Check sheet for the modelled part. Datum: model origin and axes. Units: mm. A direction names the side the tool comes from. Round coordinates to 2 decimals unless told otherwise and drop trailing zeros. Loops run counter-clockwise (first coordinate to the right, second up) from the corner with the lowest first, then second, coordinate; pieces in that order, holes last. Notation, with made-up numbers: (85, 54) - (116, 54) arc R20 ccw to (116, 74) - close; hole circle Ø1 at (2.25, 54). An arc over 180 degrees is marked (long way). Put each result on its own line as item: value. Start each with the question number.
```python
from build123d import *

# Parameters (mm, degrees)
F0_R     = 12.7
F1_DEPTH = 6.35


with BuildPart() as f1:
    # F0 (on Top) → F1 (new body)
    with BuildSketch(Plane.XY):
        with BuildLine():
            Line((22.45064, 22.45064), (37.34271, 7.55857))
            ThreePointArc((37.34271, 7.55857), (33.570952, 18.016692), (26.940768, 26.940768))
            Line((26.940768, 26.940768), (17.960512, 26.940768))
            Line((17.960512, 26.940768), (22.45064, 22.45064))
        make_face()
        with BuildLine():
            ThreePointArc((-37.34271, -7.55857), (-33.570952, -18.016692), (-26.940768, -26.940768))
            Line((-26.940768, -26.940768), (-17.960512, -26.940768))
            Line((-17.960512, -26.940768), (-22.45064, -22.45064))
            Line((-22.45064, -22.45064), (-37.34271, -7.55857))
        make_face()
        with BuildLine():
            ThreePointArc((7.159566, -37.421259), (17.657349, -33.761339), (26.651684, -27.226783))
            Line((26.651684, -27.226783), (26.747534, -18.247039))
            Line((26.747534, -18.247039), (22.209737, -22.688986))
            Line((22.209737, -22.688986), (7.159566, -37.421259))
        make_face()
        with BuildLine():
            Line((-22.45064, 22.45064), (-7.55857, 37.34271))
            ThreePointArc((-7.55857, 37.34271), (-18.016692, 33.570952), (-26.940768, 26.940768))
            Line((-26.940768, 26.940768), (-26.940768, 17.960512))
            Line((-26.940768, 17.960512), (-22.45064, 22.45064))
        make_face()
        with BuildLine():
            Line((31.75, 6.35), (38.1, 0))
            ThreePointArc((38.1, 0), (37.910205, 3.798206), (37.34271, 7.55857))
            Line((37.34271, 7.55857), (22.45064, 22.45064))
            Line((22.45064, 22.45064), (17.960512, 26.940768))
            Line((17.960512, 26.940768), (26.940768, 26.940768))
            ThreePointArc((26.940768, 26.940768), (24.120826, 29.4923), (21.060567, 31.75))
            Line((21.060567, 31.75), (0, 31.75))
            Line((0, 31.75), (-6.35, 31.75))
            Line((-6.35, 31.75), (0, 38.1))
            ThreePointArc((0, 38.1), (-3.798206, 37.910205), (-7.55857, 37.34271))
            Line((-7.55857, 37.34271), (-22.45064, 22.45064))
            Line((-22.45064, 22.45064), (-26.940768, 17.960512))
            Line((-26.940768, 17.960512), (-26.940768, 26.940768))
            ThreePointArc((-26.940768, 26.940768), (-29.4923, 24.120826), (-31.75, 21.060567))
            Line((-31.75, 21.060567), (-31.75, 0))
            Line((-31.75, 0), (-31.75, -6.35))
            Line((-31.75, -6.35), (-38.1, 0))
            ThreePointArc((-38.1, 0), (-37.910205, -3.798206), (-37.34271, -7.55857))
            Line((-37.34271, -7.55857), (-22.45064, -22.45064))
            Line((-22.45064, -22.45064), (-17.960512, -26.940768))
            Line((-17.960512, -26.940768), (-26.940768, -26.940768))
            ThreePointArc((-26.940768, -26.940768), (-24.120826, -29.4923), (-21.060567, -31.75))
            Line((-21.060567, -31.75), (0, -31.75))
            Line((0, -31.75), (6.35, -31.75))
            Line((6.35, -31.75), (0, -38.1))
            ThreePointArc((0, -38.1), (3.595834, -37.929935), (7.159566, -37.421259))
            Line((7.159566, -37.421259), (22.209737, -22.688986))
            Line((22.209737, -22.688986), (26.747534, -18.247039))
            Line((26.747534, -18.247039), (26.651684, -27.226783))
            ThreePointArc((26.651684, -27.226783), (29.363153, -24.277876), (31.75, -21.060567))
            Line((31.75, -21.060567), (31.75, 0))
            Line((31.75, 0), (31.75, 6.35))
        make_face()
        Circle(F0_R, mode=Mode.SUBTRACT)
        with BuildLine():
            ThreePointArc((31.75, -21.060567), (36.477973, -10.998523), (38.1, 0))
            Line((38.1, 0), (31.75, 6.35))
            Line((31.75, 6.35), (31.75, 0))
            Line((31.75, 0), (31.75, -21.060567))
        make_face()
        with BuildLine():
            Line((-31.75, 0), (-31.75, 21.060567))
            ThreePointArc((-31.75, 21.060567), (-36.477973, 10.998523), (-38.1, 0))
            Line((-38.1, 0), (-31.75, -6.35))
            Line((-31.75, -6.35), (-31.75, 0))
        make_face()
    extrude(amount=-F1_DEPTH)


solid = f1.part
```
Q1. Depth check by flat-ended pin: pin 1 Ø1.5 at (x, z) = (9, -3.5) entering from +Y; pin 2 Ø3 at (x, z) = (-19.5, -4) entering from +Y; pin 3 Ø1.5 at (y, z) = (-12.5, -1) entering from -X. Enter the tip coordinate at first touch or a pass-through.
Q2. Draft check along Y on faces 1 (the face through (-2.75, -12.4, -3.13)), 2 (the face through (-8, -31.75, -3)), 3 (the face through (-36.43, 11.15, -3.13)), 4 (the face through (-24.16, -29.46, -3.13)). Enter one of: +Y half, -Y half, draft (parallel to the pull), parting line (faces both ways), or undercut.
Q3. Cross-section at A-A on y = 3. Enter the section's corners in (x, z), and give its area (3 significant figures).
Q4. Cross-section at B-B on z = -3.25. Enter the section's corners in (x, y), and give its area (3 significant figures).
Q5. Cross-section at D-D on y = 20. Enter the section's corners in (x, z), and give its area (3 significant figures).
Q6. Cross-section at C-C on x = -19. Enter the section's corners in (y, z).
Q7. Material ranges on line 1 (Y direction, x = 3.5, z = -6); line 2 (Y direction, x = 7, z = -1.25); line 3 (X direction, y = 10.5, z = -5.5), recorded low to high. Write a range as from..to.
Q8. Set-up check for faces 5 (the face through (-3.2, 34.9, -3.1)), 6 (the face through (37.915, 3.745, -3.131)): record each of +Z, -Z, +X, -X, +Y, -Y from which the full face is reachable in a straight line by a thin tool's end or side.
Answer list:
1. pin 1: stops at y = 31.75
1. pin 2: stops at y = 33.58
1. pin 3: stops at x = -36.24
2. face 1: undercut
2. face 2: undercut
2. face 3: +Y half
2. face 4: -Y half
3. outline: (-37.98, -6.35) - (-12.34, -6.35) - (-12.34, 0) - (-37.98, 0) - close; (12.34, -6.35) - (37.98, -6.35) - (37.98, 0) - (12.34, 0) - close
3. area: 326 mm2
4. outline: (-38.1, 0) arc R38.1 ccw to (-37.34, -7.56) arc R38.1 ccw to (-26.94, -26.94) arc R38.1 ccw to (-21.06, -31.75) - (6.35, -31.75) - (0, -38.1) arc R38.1 ccw to (7.16, -37.42) arc R38.1 ccw to (26.65, -27.23) arc R38.1 ccw to (31.75, -21.06) arc R38.1 ccw to (38.1, 0) arc R38.1 ccw to (37.34, 7.56) arc R38.1 ccw to (26.94, 26.94) arc R38.1 ccw to (21.06, 31.75) - (-6.35, 31.75) - (0, 38.1) arc R38.1 ccw to (-7.56, 37.34) arc R38.1 ccw to (-26.94, 26.94) arc R38.1 ccw to (-31.75, 21.06) arc R38.1 ccw to start; hole circle Ø25.4 at (0, 0)
4. area: 3,830 mm2
5. outline: (-32.43, -6.35) - (32.43, -6.35) - (32.43, 0) - (-32.43, 0) - close
5. area: 412 mm2
6. outline: (-31.75, -6.35) - (33.02, -6.35) - (33.02, 0) - (-31.75, 0) - close
7. line 1: y = -37.94..-34.6, -31.75..-12.21, 12.21..31.75
7. line 2: y = -37.45..-10.6, 10.6..31.75
7. line 3: x = -36.62..-7.14, 7.14..36.62
8. face 5: +Z, -Z, +X
8. face 6: +Z, -Z, +X, +Y
